from build123d import *

# Parameters (mm, degrees)
BOSS_EXTRUDE1_DEPTH     = 19.05
CUT_EXTRUDE1_DEPTH      = 20.05
SKETCH2_4_W             = 12.954
SKETCH2_4_H             = 1.7018
CUT_EXTRUDE2_DEPTH      = 18.25625
SKETCH6_W               = 0.608326788
SKETCH6_H               = 1.5875
SKETCH8_W               = 2.576826788
SKETCH8_H               = 1.5875
SKETCH9_W               = 12.954
SKETCH9_H               = 5.08
SKETCH9_H_2             = 2.159
CUT_EXTRUDE3_DEPTH      = 6.35
SKETCH11_W              = 3.175
SKETCH11_H              = 5.08
CUT_EXTRUDE5_DEPTH      = 12.1125
CUT_EXTRUDE5_DEPTH_BACK = 12.1125
SKETCH10_R              = 1.016
CUT_EXTRUDE6_DEPTH      = 11.3505


with BuildPart() as part:
    # Sketch1 → Boss-Extrude1 (new body)
    with BuildSketch(Plane(origin=(0, 0, 0), x_dir=(1, 0, 0), z_dir=(0, 1, 0))):
        with BuildLine():
            Line((-0.79375, 9.109483901), (-0.79375, 8.535673212))
            ThreePointArc((-0.79375, 8.535673212), (-7.424002774, 4.28625), (-7.78898484, -3.580428942))
            Line((-7.78898484, -3.580428942), (-8.285919473, -3.867334286))
            ThreePointArc((-8.285919473, -3.867334286), (-7.918936292, -4.572), (-7.492169473, -5.242149615))
            Line((-7.492169473, -5.242149615), (-6.99523484, -4.95524427))
            ThreePointArc((-6.99523484, -4.95524427), (0, -8.5725), (6.99523484, -4.95524427))
            Line((6.99523484, -4.95524427), (7.492169473, -5.242149615))
            ThreePointArc((7.492169473, -5.242149615), (7.918936292, -4.572), (8.285919473, -3.867334286))
            Line((8.285919473, -3.867334286), (7.78898484, -3.580428942))
            ThreePointArc((7.78898484, -3.580428942), (7.424002774, 4.28625), (0.79375, 8.535673212))
            Line((0.79375, 8.535673212), (0.79375, 9.109483901))
            ThreePointArc((0.79375, 9.109483901), (0, 9.144), (-0.79375, 9.109483901))
        make_face()
    extrude(amount=BOSS_EXTRUDE1_DEPTH)

    # Sketch2 → Cut-Extrude1 (cut, through all)
    with BuildSketch(Plane(origin=(0, 19.05, 0), x_dir=(1, 0, 0), z_dir=(0, 1, 0))):
        with BuildLine():
            Line((-4.543615348, 4.303093955), (-3.175, 2.4638))
            Line((-3.175, 2.4638), (3.175, 2.4638))
            Line((3.175, 2.4638), (4.543615348, 4.303093955))
            ThreePointArc((4.543615348, 4.303093955), (4.598203733, 4.928342625), (4.064, 5.2578))
            Line((4.064, 5.2578), (-4.064, 5.2578))
            ThreePointArc((-4.064, 5.2578), (-4.598203733, 4.928342625), (-4.543615348, 4.303093955))
        make_face()
    extrude(amount=-CUT_EXTRUDE1_DEPTH, mode=Mode.SUBTRACT)

    # Sketch2_4 → Cut-Extrude2 (cut)
    with BuildSketch(Plane(origin=(0, 19.05, 0), x_dir=(1, 0, 0), z_dir=(0, 1, 0))):
        with Locations((0, 1.6129)):
            Rectangle(SKETCH2_4_W, SKETCH2_4_H)
    extrude(amount=-CUT_EXTRUDE2_DEPTH, mode=Mode.SUBTRACT)

    # Sketch6 → Cut-Revolve2 (revolve, cut)
    with BuildSketch(Plane(origin=(0, 0, 0), x_dir=(0, 0, -1), z_dir=(1, 0, 0))):
        with Locations((8.839836606, 0.79375)):
            Rectangle(SKETCH6_W, SKETCH6_H)
    revolve(axis=Axis((0, 19.730213777, 0), (0, -1, 0)), mode=Mode.SUBTRACT)

    # Sketch8 → Revolve2 (revolve)
    with BuildSketch(Plane(origin=(0, 0, 0), x_dir=(0, 0, -1), z_dir=(1, 0, 0))):
        with Locations((9.824086606, 0.79375)):
            Rectangle(SKETCH8_W, SKETCH8_H)
    revolve(axis=Axis((0, 4.48386458, 0), (0, -1, 0)))

    # Sketch9 → Cut-Extrude3 (cut)
    with BuildSketch(Plane(origin=(0, 19.05, 0), x_dir=(1, 0, 0), z_dir=(0, 1, 0))):
        with Locations((0, -1.778)):
            Rectangle(SKETCH9_W, SKETCH9_H)
        with Locations((0, 3.5433)):
            Rectangle(SKETCH9_W, SKETCH9_H_2)
    extrude(amount=-CUT_EXTRUDE3_DEPTH, mode=Mode.SUBTRACT)

    # Sketch11 → Cut-Extrude5 (cut, two sides)
    with BuildSketch(Plane(origin=(0, 0, 0), x_dir=(0, 0, -1), z_dir=(1, 0, 0))) as cut_extrude5_sk:
        with Locations((7.5565, 7.77875)):
            Rectangle(SKETCH11_W, SKETCH11_H)
    extrude(amount=CUT_EXTRUDE5_DEPTH, mode=Mode.SUBTRACT)
    extrude(cut_extrude5_sk.sketch, amount=-CUT_EXTRUDE5_DEPTH_BACK, mode=Mode.SUBTRACT)

    # Sketch10 → Cut-Extrude6 (cut, through all)
    with BuildSketch(Plane(origin=(0, 0, -0.762), x_dir=(-1, 0, 0), z_dir=(0, 0, -1))):
        with Locations((-4.572, 7.39775)):
            Circle(SKETCH10_R)
        with Locations((4.445, 7.39775)):
            Circle(SKETCH10_R)
    extrude(amount=CUT_EXTRUDE6_DEPTH, mode=Mode.SUBTRACT)


solid = part.part
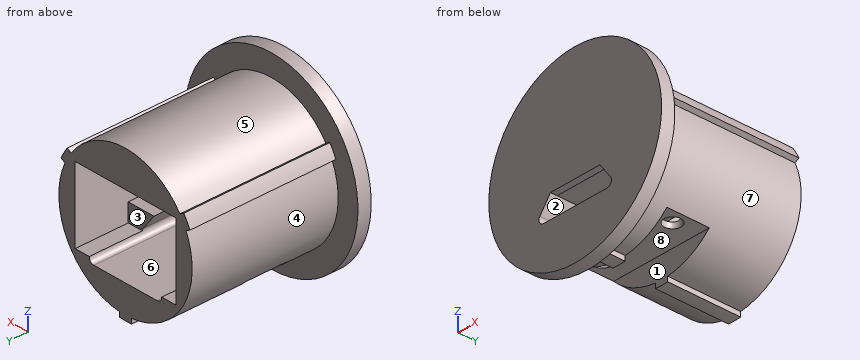
Design review of the part built by this model. Coordinates are the model's own, in mm. Face numbers are marked on the shaded views. A direction names the side the tool comes from. Give positions to 0.01 mm unless a question says otherwise; leave off trailing zeros. Write each loop counter-clockwise with the first axis right and the second up, starting at its lowest first coordinate (ties: lowest second). Pieces come first, ordered by that corner, then holes. Notation, with made-up numbers: M -30,3.5 L -20,3.5 A15 ccw -20,30.5 Z; hole C 18.5,71 d6. An arc over 180 degrees is marked long. Answer as a JSON object with one key per item and string values. Group by question number.
1) We need section A-A (x = 0). Give the boundary of the cut face in (y, z).
2) We need section B-B (y = 2.75). Give the boundary of the cut face in (x, z) (1 decimal), and give its area (3 significant figures).
3) We need section C-C (z = -6.75). Give the boundary of the cut face in (x, y), and give its area (3 significant figures).
4) Mouldability with a two-part tool opening along X and no side actions: class the marked faces 6, 7 and 8 as released by +X, released by -X, zero draft, split by the parting line, or undercut.
5) We need section D-D (z = 0). Give the boundary of the cut face in (x, y), and give its area (3 significant figures).
6) For line 1 along Z through (x, y) = (-3.5, 11.75); line 2 along Y through (x, z) = (5, 3.25); line 3 along X through (y, z) = (9.5, -2.75), list the stretches that pass through material, from the lowest coordinate up.
7) Tool access review of the marked faces 1, 2, 3, 4 and 5: name each direction out of +Z, -Z, +X, -X, +Y, -Y from which nothing blocks a thin tool from reaching the whole face with its end or side.
8) Clearance check with flat-ended pins moving along their axes: pin 1 Ø2 at (y, z) = (5.5, -0.5) entering from -X; pin 2 Ø6 at (x, z) = (-0.5, 0) entering from +Y; pin 3 Ø7 at (y, z) = (13.5, 0) entering from +X; pin 4 Ø10 at (x, z) = (3, 6.5) entering from -Y. State where each tip first meets the part, or that it passes through.
Answer key:
{
 "1": {"outline": "M 0,-11.11 L 1.59,-11.11 L 1.59,-9.14 L 5.24,-9.14 L 5.24,-5.97 L 10.32,-5.97 L 10.32,-9.14 L 19.05,-9.14 L 19.05,-5.26 L 0,-5.26 Z; M 0,-2.46 L 0.79,-2.46 L 0.79,-0.76 L 12.7,-0.76 L 12.7,4.32 L 19.05,4.32 L 19.05,8.57 L 1.59,8.57 L 1.59,11.11 L 0,11.11 Z"},
 "2": {"outline": "M -8.3,3.9 L -7.8,3.6 A8.6 ccw -0.8,-8.5 L -0.8,-9.1 A9.1 ccw 0.8,-9.1 L 0.8,-8.5 A8.6 ccw 7.8,3.6 L 8.3,3.9 A9.1 ccw 7.5,5.2 L 7,5 A8.6 ccw -7,5 L -7.5,5.2 A9.1 ccw Z; hole M -6.5,-2.5 L -3.2,-2.5 L -4.5,-4.3 A0.6 ccw -4.1,-5.3 L 4.1,-5.3 A0.6 ccw 4.5,-4.3 L 3.2,-2.5 L 6.5,-2.5 L 6.5,-0.8 L -6.5,-0.8 Z", "area": "189 mm²"},
 "3": {"outline": "M -8.83,0 L 8.83,0 L 8.83,1.59 L 5.28,1.59 L 5.28,5.24 L -5.28,5.24 L -5.28,1.59 L -8.83,1.59 Z; M -5.28,10.32 L 5.28,10.32 L 5.28,19.05 L -5.28,19.05 Z", "area": "159 mm²"},
 "4": {"face 6": "undercut", "face 7": "released by +X", "face 8": "zero draft"},
 "5": {"outline": "M -11.11,0 L 11.11,0 L 11.11,1.59 L 8.57,1.59 L 8.57,19.05 L 6.48,19.05 L 6.48,12.7 L -6.48,12.7 L -6.48,19.05 L -8.57,19.05 L -8.57,1.59 L -11.11,1.59 Z", "area": "252 mm²"},
 "6": {"line 1": "z = -7.83 to -5.26, -2.9 to -2.46, -0.76 to 7.83", "line 2": "y = 0 to 12.7", "line 3": "x = -8.12 to -3.39, 3.39 to 8.12"},
 "7": {"face 1": "-Z, +X, -X", "face 2": "+Y, -Y", "face 3": "+Y", "face 4": "-X, +Y", "face 5": "+Z, +Y"},
 "8": {"pin 1": "stops at x = -8.57", "pin 2": "stops at y = 12.7", "pin 3": "stops at x = 8.57", "pin 4": "stops at y = 0"}
}
